from build123d import *

# Parameters (mm, degrees)
SKETCH1_W           = 50.8
SKETCH1_H           = 82.55
BOSS_EXTRUDE1_DEPTH = 3.175
FILLET1_R           = 2.54
SKETCH2_R           = 2.54
CUT_EXTRUDE1_DEPTH  = 4.175
SKETCH2_2_R         = 2.54
BOSS_EXTRUDE2_DEPTH = 3.175
SKETCH3_R           = 0.9525
CUT_EXTRUDE2_DEPTH  = 4.175


with BuildPart() as part:
    # Sketch1 → Boss-Extrude1 (new body)
    with BuildSketch(Plane(origin=(0, 0, 0), x_dir=(1, 0, 0), z_dir=(0, 1, 0))):
        with Locations((25.4, -41.275)):
            Rectangle(SKETCH1_W, SKETCH1_H)
    extrude(amount=BOSS_EXTRUDE1_DEPTH)

    # Fillet1
    fillet1_edges = [part.edges().sort_by_distance(p)[0] for p in [
        (50.8, 3.175, 41.275),
        (25.4, 3.175, 0),
        (0, 3.175, 41.275),
        (25.4, 3.175, 82.55),
        (0, 1.5875, 0),
        (50.8, 1.5875, 0),
        (50.8, 1.5875, 82.55),
        (0, 1.5875, 82.55),
    ]]
    fillet(fillet1_edges, radius=FILLET1_R)

    # Sketch2 → Cut-Extrude1 (cut, through all)
    with BuildSketch(Plane(origin=(0, 3.175, 0), x_dir=(1, 0, 0), z_dir=(0, 1, 0))):
        with Locations((48.26, -80.01)):
            Circle(SKETCH2_R)
        with Locations((2.54, -80.01)):
            Circle(SKETCH2_R)
        with Locations((2.54, -2.54)):
            Circle(SKETCH2_R)
        with Locations((48.26, -2.54)):
            Circle(SKETCH2_R)
    extrude(amount=-CUT_EXTRUDE1_DEPTH, mode=Mode.SUBTRACT)

    # Sketch2<2> → Boss-Extrude2 (add)
    with BuildSketch(Plane(origin=(0, 3.175, 0), x_dir=(1, 0, 0), z_dir=(0, 1, 0))):
        with Locations((48.26, -80.01)):
            Circle(SKETCH2_2_R)
        with Locations((2.54, -80.01)):
            Circle(SKETCH2_2_R)
        with Locations((2.54, -2.54)):
            Circle(SKETCH2_2_R)
        with Locations((48.26, -2.54)):
            Circle(SKETCH2_2_R)
    extrude(amount=-BOSS_EXTRUDE2_DEPTH)

    # Sketch3 → Cut-Extrude2 (cut, through all)
    with BuildSketch(Plane(origin=(0, 3.175, 0), x_dir=(1, 0, 0), z_dir=(0, 1, 0))):
        with Locations((2.54, -2.54)):
            Circle(SKETCH3_R)
        with Locations((48.26, -2.54)):
            Circle(SKETCH3_R)
        with Locations((2.54, -80.01)):
            Circle(SKETCH3_R)
        with Locations((48.26, -80.01)):
            Circle(SKETCH3_R)
    extrude(amount=-CUT_EXTRUDE2_DEPTH, mode=Mode.SUBTRACT)


solid = part.part
Work out the finished part from the listing and answer in its coordinate system (mm). A direction names the side the tool comes from. Round coordinates to 2 decimals unless told otherwise and drop trailing zeros. Loops run counter-clockwise (first coordinate to the right, second up) from the corner with the lowest first, then second, coordinate; pieces in that order, holes last. Notation, with made-up numbers: (55.5, -12) - (114.5, -12) arc R22 cw to (114.5, 4) - close; hole circle Ø2 at (-18.5, 45). An arc over 180 degrees is marked (long way). Use one line per item in the form item = value. Start each with the question number.
(1) Find section B-B on z = 59. Determine the outline of the cut face in (x, y) (3 decimals), and give its area (3 significant figures).
(2) Determine the mould class of faces 1 (the face through (25, 3.175, 41)), 2 (the face through (1.59, 1.61, 2.5)), 3 (the face through (50.076, 2.411, 40.733)) for opening direction X: +X half, -X half, draft (parallel to the pull), parting line (faces both ways), or undercut.
(3) Flat-ended cylindrical pins translate along their axes: P1, Ø1.5, axis at x = 42, y = 2, coming from the +Z side; P2, Ø1, axis at y = 3, z = 12, coming from the +X side. Find the tip coordinate at first contact, or state that the pin passes through.
(4) Consider line 1 (X direction, y = 0.9, z = 80.01); line 2 (Z direction, x = 2.54, y = 0.8); line 3 (Z direction, x = 46, y = 0.9). Determine where each line is inside the solid, lowest interval first.
(5) Find section A-A on y = 2.35. Determine the outline of the cut face in (x, z) (1 decimal).
(6) Which of the six approach directions +Z, -Z, +X, -X, +Y, -Y give full straight-line access (tool end or side, diameter ignored) to faces 4 (the face through (0.724, 2.411, 40.733)), 5 (the face through (50, 1.96, 81.86)), 6 (the face through (2.416, 1.61, 79.066)), 7 (the face through (25.72, 2.411, 81.826)), 8 (the face through (25.72, 2.411, 0.724))?
Answer list:
q1.outline = (0, 0) - (50.8, 0) - (50.8, 0.635) arc R2.54 ccw to (48.26, 3.175) - (2.54, 3.175) arc R2.54 ccw to (0, 0.635) - close
q1.area = 159 mm^2
q2.face_1 = draft
q2.face_2 = undercut
q2.face_3 = +X half
q3.P1 = 82.47
q3.P2 = 49.98
q4.line_1 = 0 to 1.59, 3.49 to 47.31, 49.21 to 50.8
q4.line_2 = 0 to 1.59, 3.49 to 79.06, 80.96 to 82.55
q4.line_3 = 0.01 to 82.54
q5.outline = (0.7, 4.3) arc R2.5 ccw to (4.3, 0.7) - (46.5, 0.7) arc R2.5 ccw to (50.1, 4.3) - (50.1, 78.3) arc R2.5 ccw to (46.5, 81.9) - (4.3, 81.9) arc R2.5 ccw to (0.7, 78.3) - close; hole circle Ø1.9 at (2.5, 2.5); hole circle Ø1.9 at (2.5, 80); hole circle Ø1.9 at (48.3, 2.5); hole circle Ø1.9 at (48.3, 80)
q6.face_4 = -X, +Y
q6.face_5 = +Y
q6.face_6 = +Y, -Y
q6.face_7 = +Z, +Y
q6.face_8 = -Z, +Y
